Read the model definition and answer for the solid it produces. Units are mm, in the model's axes. Face numbers are marked on the shaded views. A direction names the side the tool comes from. Coordinates: 2 decimals unless noted, no trailing zeros. Write each loop counter-clockwise with the first axis right and the second up, starting at its lowest first coordinate (ties: lowest second). Pieces come first, ordered by that corner, then holes. Notation, with made-up numbers: (89.25, 66.5) -> (104.25, 66.5) arc R30 ccw to (104.25, 91.5) -> close; hole circle Ø4 at (21, 72.5). An arc over 180 degrees is marked (long way). Write item = value, one per line. Start each with the question number.
1) Find the intervals of material crossed by line 1 along Y through (x, z) = (0, 2.1); line 2 along Y through (x, z) = (7.5, 4.05); line 3 along Y through (x, z) = (2, -18), in increasing order. Write a range as from..to.
2) Section D-D (z = -29.5) is taken. Determine the outline of the cut face in (x, y).
3) Section C-C (y = 6) is taken. Determine the outline of the cut face in (x, z).
4) Flat-ended cylindrical pins translate along their axes: pin 1 Ø4 at (x, z) = (9.5, -37.5) entering from -Y; pin 2 Ø5 at (x, y) = (0, 14) entering from +Z; pin 3 Ø1.5 at (x, y) = (-12, 2) entering from -Z; pin 4 Ø15 at (x, z) = (3.5, -16.5) entering from +Y. Find the tip coordinate at first contact, or state that the pin passes through.
5) Section B-B (y = -1) is taken. Determine the outline of the cut face in (x, z), plus the area to 3 significant figures.
6) Section A-A (x = 0) is taken. Determine the outline of the cut face in (y, z).
7) A tool of negligible diameter and unlimited length cuts with its end or side. For the marked faces 1 and 2, from which of +Z, -Z, +X, -X, +Y, -Y can it reach the whole face along a straight path? Write none if from no direction.
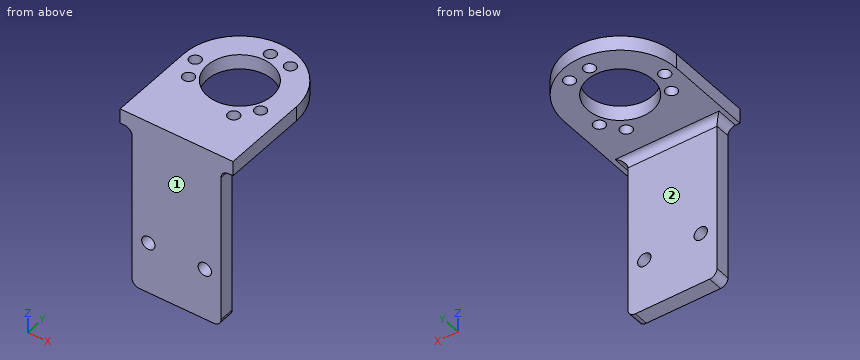
from build123d import *

# Parameters (mm, degrees)
SKETCH1_R            = 19
SKETCH1_R_2          = 11
BOSS_EXTRUDE1_DEPTH  = 5
SKETCH2_W            = 30
SKETCH2_H            = 5
BOSS_EXTRUDE2_DEPTH  = 55
M3_CLEARANCE_HOLE1_D = 3.9
M4_CLEARANCE_HOLE1_D = 4.5
FILLET1_R            = 2.5


with BuildPart() as part:
    # Sketch1 → Boss-Extrude1 (new body)
    # profile 1 of 2: a face of its own
    with BuildSketch(Plane.XY):
        Circle(SKETCH1_R)
        Circle(SKETCH1_R_2, mode=Mode.SUBTRACT)
    # profile 2 of 2: a face of its own
    with BuildSketch(Plane.XY):
        with BuildLine():
            ThreePointArc((19, 0), (0, -19), (-19, 0))
            Line((-19, 0), (-19, -29))
            Line((-19, -29), (19, -29))
            Line((19, -29), (19, 0))
        make_face()
    extrude(amount=BOSS_EXTRUDE1_DEPTH)

    # Sketch2 → Boss-Extrude2 (add)
    with BuildSketch(Plane(origin=(0, 0, 0), x_dir=(-1, 0, 0), z_dir=(0, 0, -1))):
        with Locations((0, -26.5)):
            Rectangle(SKETCH2_W, SKETCH2_H)
    extrude(amount=BOSS_EXTRUDE2_DEPTH)

    # M3 Clearance Hole1 (through all)
    with Locations(Plane.XY.offset(5)):
        with Locations((-15, 0), (0, 14), (12.124355653, -7), (-12.124355653, -7), (7.5, 12.990381057), (7.5, -12.990381057)):
            Hole(M3_CLEARANCE_HOLE1_D / 2)

    # M4 Clearance Hole1 (through all)
    with Locations(Plane(origin=(0, -24, 0), x_dir=(1, 0, 0), z_dir=(0, 1, 0))):
        with Locations((-9.5, 37.5), (9.5, 37.5)):
            Hole(M4_CLEARANCE_HOLE1_D / 2)

    # Fillet1
    fillet1_edges = [part.edges().sort_by_distance(p)[0] for p in [
        (15, -26.5, 0),
        (-15, -26.5, 0),
        (0, -24, 0),
        (15, -26.5, -55),
        (-15, -26.5, -55),
    ]]
    fillet(fillet1_edges, radius=FILLET1_R)


solid = part.part
Answer key:
q1.line_1 = -29..-11, 11..12.05, 15.95..19
q1.line_2 = -29..-14.94, -11.04..-8.05, 8.05..11.04, 14.94..17.46
q1.line_3 = -29..-24
q2.outline = (-15, -29) -> (15, -29) -> (15, -24) -> (-15, -24) -> close
q3.outline = (-18.03, 0) -> (-9.22, 0) -> (-9.22, 5) -> (-18.03, 5) -> close; (9.22, 0) -> (18.03, 0) -> (18.03, 5) -> (9.22, 5) -> close
q4.pin_1 = through
q4.pin_2 = 5
q4.pin_3 = 0
q4.pin_4 = -24
q5.outline = (-19, 0) -> (-16.67, 0) -> (-16.67, 5) -> (-19, 5) -> close; (-13.33, 0) -> (-10.95, 0) -> (-10.95, 5) -> (-13.33, 5) -> close; (10.95, 0) -> (19, 0) -> (19, 5) -> (10.95, 5) -> close
q5.area = 63.7 mm^2
q6.outline = (-29, -55) -> (-24, -55) -> (-24, -2.5) arc R2.5 cw to (-21.5, 0) -> (-11, 0) -> (-11, 5) -> (-29, 5) -> close; (11, 0) -> (12.05, 0) -> (12.05, 5) -> (11, 5) -> close; (15.95, 0) -> (19, 0) -> (19, 5) -> (15.95, 5) -> close
q7.face_1 = +Z, -Z, +X, -X, -Y
q7.face_2 = -Z, +X, -X, +Y
